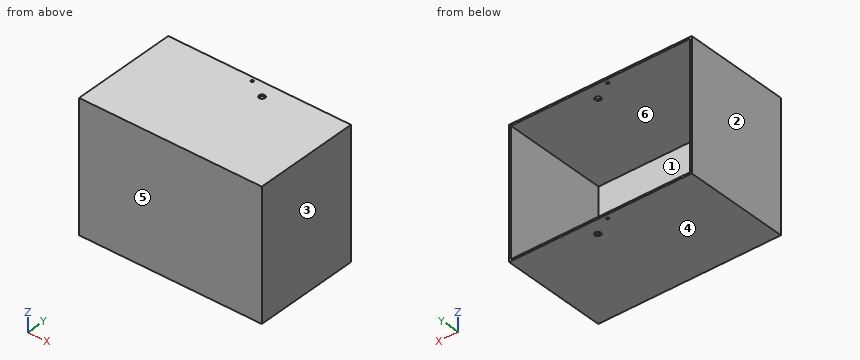
from build123d import *

# Parameters (mm, degrees)
SKETCH1_W               = 298.45
SKETCH1_H               = 209.55
BOSS_EXTRUDE1_DEPTH     = 3.175
SKETCH1_3_W             = 304.8
SKETCH1_3_H             = 215.9
SKETCH1_3_W_2           = 298.45
SKETCH1_3_H_2           = 209.55
BOSS_EXTRUDE2_DEPTH     = 177.8
SKETCH2_R               = 4.953
SKETCH2_R_2             = 2.15
CUT_EXTRUDE1_DEPTH      = 1
CUT_EXTRUDE1_DEPTH_BACK = 216.9


with BuildPart() as part:
    # Sketch1 → Boss-Extrude1 (new body)
    with BuildSketch(Plane(origin=(0, 0, 0), x_dir=(1, 0, 0), z_dir=(0, 1, 0))):
        Rectangle(SKETCH1_W, SKETCH1_H)
    extrude(amount=BOSS_EXTRUDE1_DEPTH)

    # Sketch1<3> → Boss-Extrude2 (add)
    with BuildSketch(Plane(origin=(0, 0, 0), x_dir=(1, 0, 0), z_dir=(0, 1, 0))):
        Rectangle(SKETCH1_3_W, SKETCH1_3_H)
        Rectangle(SKETCH1_3_W_2, SKETCH1_3_H_2, mode=Mode.SUBTRACT)
    extrude(amount=BOSS_EXTRUDE2_DEPTH)

    # Sketch2 → Cut-Extrude1 (cut, two sides)
    with BuildSketch(Plane.XY.offset(107.95)) as cut_extrude1_sk:
        with Locations((25.4, 152.4)):
            Circle(SKETCH2_R)
        with Locations((-6.35, 170.7322)):
            Circle(SKETCH2_R_2)
    extrude(amount=CUT_EXTRUDE1_DEPTH, mode=Mode.SUBTRACT)
    extrude(cut_extrude1_sk.sketch, amount=-CUT_EXTRUDE1_DEPTH_BACK, mode=Mode.SUBTRACT)


solid = part.part
Verification items for the finished model (mm, model axes). Face numbers are marked on the shaded views. A direction names the side the tool comes from. Coordinates: 2 decimals unless noted, no trailing zeros. Order: outer loops, then holes, each group sorted by start corner. A loop starts at its lowest first (then second) coordinate and runs counter-clockwise, first axis right, second up.
Item 1: Depth check by flat-ended pin: pin 1 (12 mm diameter, centred on x = 43, z = 41.5, fed in from +Y) (3 decimals). Enter the tip coordinate at first touch or a pass-through.
Filled in:
pin 1: stops at y = 3.175
Item 2: Section check B-B, the plane z = -46. Enter the section's corners in (x, y) (3 decimals).
Filled in:
outline: (-152.4, 0) - (152.4, 0) - (152.4, 177.8) - (149.225, 177.8) - (149.225, 3.175) - (-149.225, 3.175) - (-149.225, 177.8) - (-152.4, 177.8) - close
Item 3: Material ranges on L1, parallel to Z at x = -134.5, y = 19 (3 decimals); L2, parallel to X at y = 64.5, z = -79 (3 decimals); L3, parallel to Y at x = -6, z = -105, recorded low to high.
Filled in:
L1: z = -107.95 to -104.775, 104.775 to 107.95
L2: x = -152.4 to -149.225, 149.225 to 152.4
L3: y = 0 to 168.61, 172.85 to 177.8
Item 4: Release check for a two-part mould opening along X. For the marked faces 1, 2, 3 and 4 record: +X half, -X half, draft (parallel to the pull), parting line (faces both ways), or undercut.
Filled in:
face 1: undercut
face 2: -X half
face 3: +X half
face 4: draft
Item 5: Section check C-C, the plane y = 20. Enter the section's corners in (x, z) (3 decimals).
Filled in:
outline: (-152.4, -107.95) - (152.4, -107.95) - (152.4, 107.95) - (-152.4, 107.95) - close; hole (-149.225, -104.775) - (149.225, -104.775) - (149.225, 104.775) - (-149.225, 104.775) - close
Item 6: Section check D-D, the plane x = 89.5. Enter the section's corners in (y, z) (3 decimals), then the cut area to 3 significant figures.
Filled in:
outline: (0, -107.95) - (177.8, -107.95) - (177.8, -104.775) - (3.175, -104.775) - (3.175, 104.775) - (177.8, 104.775) - (177.8, 107.95) - (0, 107.95) - close
area: 1,790 mm2
Item 7: Access from +Z, -Z, +X, -X, +Y, -Y to the whole of each face (thin tool, end or side, straight path). Record for the marked faces 5 and 6.
Filled in:
face 5: +Z, -Z, +X, -X, -Y
face 6: +Y
Item 8: Section check A-A, the plane x = 25.4. Enter the section's corners in (y, z) (3 decimals), then the cut area to 3 significant figures.
Filled in:
outline: (0, -107.95) - (147.447, -107.95) - (147.447, -104.775) - (3.175, -104.775) - (3.175, 104.775) - (147.447, 104.775) - (147.447, 107.95) - (0, 107.95) - close; (157.353, -107.95) - (177.8, -107.95) - (177.8, -104.775) - (157.353, -104.775) - close; (157.353, 104.775) - (177.8, 104.775) - (177.8, 107.95) - (157.353, 107.95) - close
area: 1,730 mm2
